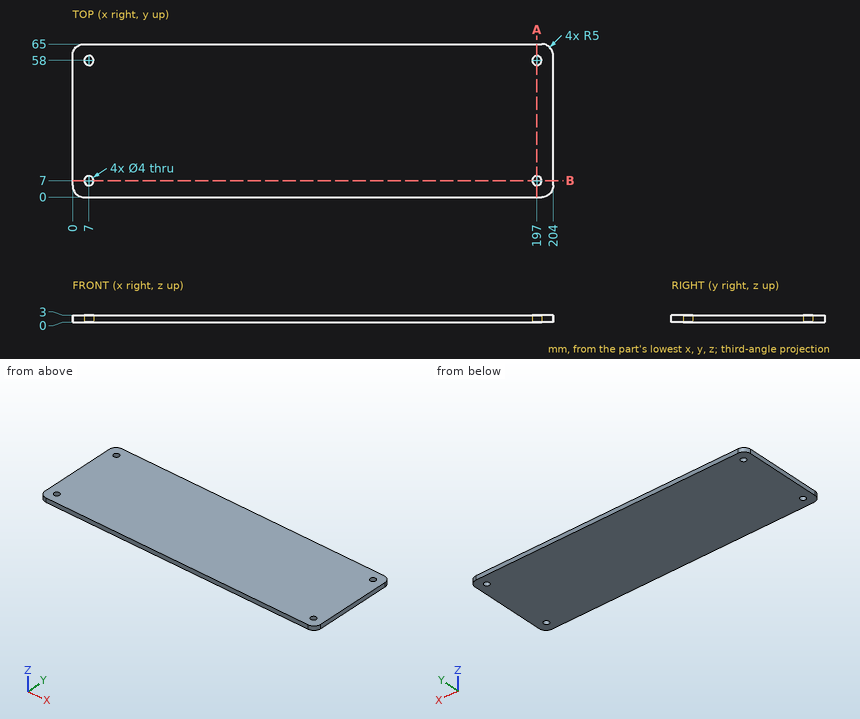
Source: three-view drawing plus pictorial views. Frame: mm from the lowest corner of the part. Round coordinates to 2 decimals unless told otherwise and drop trailing zeros. Loops run counter-clockwise (first coordinate to the right, second up) from the corner with the lowest first, then second, coordinate; pieces in that order, holes last.
Q1. Section B-B, the plane y = 7. Return loops of the section in (x, z).
Q2. Ray query, line 1 (Y direction, x = 197, z = 1.15); line 2 (X direction, y = 57, z = 1.3). Return the intervals inside material, ascending.
Q3. First-contact query: P1, Ø4.5, axis at x = 7, y = 58, coming from the +Z side. Flat tip, straight axial feed; report the tip coordinate or a pass-through.
Q4. Section A-A, the plane x = 197. Return loops of the section in (y, z).
Solutions:
1. outline: (0, 0) - (5, 0) - (5, 3) - (0, 3) - close; (9, 0) - (195, 0) - (195, 3) - (9, 3) - close; (199, 0) - (204, 0) - (204, 3) - (199, 3) - close
2. line 1: y = 0 to 5, 9 to 56, 60 to 65
2. line 2: x = 0 to 5.27, 8.73 to 195.27, 198.73 to 204
3. P1: stops at z = 3
4. outline: (0, 0) - (5, 0) - (5, 3) - (0, 3) - close; (9, 0) - (56, 0) - (56, 3) - (9, 3) - close; (60, 0) - (65, 0) - (65, 3) - (60, 3) - close
